```python
from build123d import *

# Parameters (mm, degrees)
SKETCH1_W           = 127
SKETCH1_H           = 127
BOSS_EXTRUDE1_DEPTH = 18
SKETCH2_W           = 127
SKETCH2_H           = 19
CUT_EXTRUDE1_DEPTH  = 6.35
SKETCH3_W           = 18.5
SKETCH3_H           = 127
CUT_EXTRUDE2_DEPTH  = 6.35


with BuildPart() as part:
    # Sketch1 → Boss-Extrude1 (new body)
    with BuildSketch(Plane(origin=(0, 0, 0), x_dir=(1, 0, 0), z_dir=(0, 1, 0))):
        Rectangle(SKETCH1_W, SKETCH1_H)
    extrude(amount=BOSS_EXTRUDE1_DEPTH)

    # Sketch2 → Cut-Extrude1 (cut)
    with BuildSketch(Plane(origin=(0, 18, 0), x_dir=(1, 0, 0), z_dir=(0, 1, 0))):
        with Locations((0, -15.9)):
            Rectangle(SKETCH2_W, SKETCH2_H)
    extrude(amount=-CUT_EXTRUDE1_DEPTH, mode=Mode.SUBTRACT)

    # Sketch3 → Cut-Extrude2 (cut)
    with BuildSketch(Plane(origin=(0, 18, 0), x_dir=(1, 0, 0), z_dir=(0, 1, 0))):
        with Locations((54.25, 0)):
            Rectangle(SKETCH3_W, SKETCH3_H)
        with Locations((-54.25, 0)):
            Rectangle(SKETCH3_W, SKETCH3_H)
    extrude(amount=-CUT_EXTRUDE2_DEPTH, mode=Mode.SUBTRACT)


solid = part.part
```
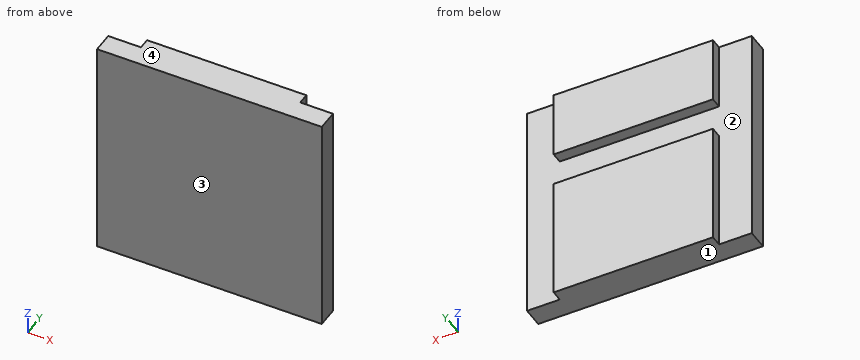
Model file for the job. Use its own axes, mm. Face numbers are marked on the shaded views. Coordinates: 2 decimals unless noted, no trailing zeros. Write each loop counter-clockwise with the first axis right and the second up, starting at its lowest first coordinate (ties: lowest second). Pieces come first, ordered by that corner, then holes. Notation, with made-up numbers: (77, 28.25) - (107, 28.25) arc R16 ccw to (107, 58.25) - close; hole circle Ø3 at (71.25, -39). An arc over 180 degrees is marked (long way). One line per question, with ' | ' between items. Start each with the question number.
Q1. Pin check, flat tips, straight feed: pin 1 (3 mm diameter, centred on y = 15, z = -19.5, fed in from -X); pin 2 (1.9 mm diameter, centred on y = 14.5, z = 53, fed in from +X). Stop position of each tip, or through.
Q2. Cut at A-A, the plane y = 13.5. List the corners of the cut face in (x, z).
Q3. Pull direction Z, two halves, no side cores. Call the marked faces 1, 2, 3 and 4: pulls with the +Z half, pulls with the -Z half, needs draft (parallel to the pull), parting line crosses it, or undercut.
Q4. Cut at D-D, the plane z = 20.5. List the corners of the cut face in (x, y).
Q5. Cut at B-B, the plane z = 46.5. List the corners of the cut face in (x, y).
Q6. Cut at C-C, the plane x = 11. List the corners of the cut face in (y, z).
Q7. Drill centre lines: line 1 (Z direction, x = 19.5, y = 15); line 2 (Y direction, x = 55, z = -27.5); line 3 (X direction, y = 14, z = -16.5). Where is each one in solid material? Low to high. Write a range as [from, to].
Answer below:
1) pin 1: x = -45 | pin 2: x = 45
2) outline: (-45, -63.5) - (45, -63.5) - (45, 6.4) - (-45, 6.4) - close; (-45, 25.4) - (45, 25.4) - (45, 63.5) - (-45, 63.5) - close
3) face 1: pulls with the -Z half | face 2: undercut | face 3: needs draft | face 4: pulls with the +Z half
4) outline: (-63.5, 0) - (63.5, 0) - (63.5, 11.65) - (-63.5, 11.65) - close
5) outline: (-63.5, 0) - (63.5, 0) - (63.5, 11.65) - (45, 11.65) - (45, 18) - (-45, 18) - (-45, 11.65) - (-63.5, 11.65) - close
6) outline: (0, -63.5) - (18, -63.5) - (18, 6.4) - (11.65, 6.4) - (11.65, 25.4) - (18, 25.4) - (18, 63.5) - (0, 63.5) - close
7) line 1: [-63.5, 6.4], [25.4, 63.5] | line 2: [0, 11.65] | line 3: [-45, 45]
